from build123d import *

# Parameters (mm, degrees)
SKETCH1_R           = 5
BOSS_EXTRUDE1_DEPTH = 20
SKETCH2_R           = 5
CUT_EXTRUDE1_DEPTH  = 75
SKETCH3_R           = 22.485447426
BOSS_EXTRUDE2_DEPTH = 3.5
SKETCH4_R           = 20.327044556
BOSS_EXTRUDE3_DEPTH = 5.5
SKETCH5_R           = 18.043078954
SKETCH5_R_2         = 5.853514337
CUT_EXTRUDE2_DEPTH  = 2
BOSS_EXTRUDE5_START = 25
SKETCH7_R           = 5.853514337
BOSS_EXTRUDE5_DEPTH = 25


with BuildPart() as part:
    # Sketch1 → Boss-Extrude1 (new body)
    with BuildSketch(Plane(origin=(0, 0, 0), x_dir=(1, 0, 0), z_dir=(0, 1, 0))):
        with BuildLine():
            Line((9.177252883, 11.533668593), (42.143741373, -0.928512909))
            ThreePointArc((42.143741373, -0.928512909), (70.658147952, -5.539619318), (42.614104982, -12.458097383))
            Line((42.614104982, -12.458097383), (7.783972854, -12.458097383))
            ThreePointArc((7.783972854, -12.458097383), (-1.224173666, -20.477404202), (-9.243480486, -11.469257682))
            Line((-9.243480486, -11.469257682), (-23.565055604, -11.469257682))
            ThreePointArc((-23.565055604, -11.469257682), (-58.758292474, 4.433528189), (-20.995467888, 12.522508294))
            Line((-20.995467888, 12.522508294), (-7.850200457, 12.522508294))
            ThreePointArc((-7.850200457, 12.522508294), (1.157946064, 20.541815114), (9.177252883, 11.533668593))
        make_face()
        with Locations(Location((0.663526213, 12.028088444, 0), (0, 0, 270))):
            Circle(SKETCH1_R, mode=Mode.SUBTRACT)
        with Locations(Location((-0.729753816, -11.963677532, 0), (0, 0, 270))):
            Circle(SKETCH1_R, mode=Mode.SUBTRACT)
    extrude(amount=BOSS_EXTRUDE1_DEPTH)

    # Sketch2 → Cut-Extrude1 (cut)
    with BuildSketch(Plane(origin=(0, 20, 0), x_dir=(1, 0, 0), z_dir=(0, 1, 0))):
        with Locations(Location((55.93095175, -6.140433438, 0), (0, 0, 270))):
            Circle(SKETCH2_R)
    extrude(amount=-CUT_EXTRUDE1_DEPTH, mode=Mode.SUBTRACT)

    # Sketch3 → Boss-Extrude2 (add)
    with BuildSketch(Plane.XZ):
        with Locations(Location((-38.546840471, -2.268823063, 0), (0, 0, 37.660146308))):
            Circle(SKETCH3_R)
    extrude(amount=BOSS_EXTRUDE2_DEPTH)

    # Sketch4 → Boss-Extrude3 (add)
    with BuildSketch(Plane(origin=(0, 20, 0), x_dir=(1, 0, 0), z_dir=(0, 1, 0))):
        with Locations(Location((-38.546840471, 2.268823063, 0), (0, 0, 30.293894425))):
            Circle(SKETCH4_R)
    extrude(amount=BOSS_EXTRUDE3_DEPTH)

    # Sketch5 → Cut-Extrude2 (cut)
    with BuildSketch(Plane.XZ.offset(3.5)):
        with Locations(Location((-38.546840471, -2.268823063, 0), (0, 0, 270))):
            Circle(SKETCH5_R)
        with Locations(Location((-38.546840471, -2.268823063, 0), (0, 0, 270))):
            Circle(SKETCH5_R_2, mode=Mode.SUBTRACT)
    extrude(amount=-CUT_EXTRUDE2_DEPTH, mode=Mode.SUBTRACT)

    # Sketch7 → Boss-Extrude5 (add)
    with BuildSketch(Plane.XZ.offset(3.5).offset(BOSS_EXTRUDE5_START)):
        with Locations(Location((-38.546840471, -2.268823063, 0), (0, 0, 270))):
            Circle(SKETCH7_R)
    extrude(amount=-BOSS_EXTRUDE5_DEPTH)


solid = part.part
The model under review builds one solid part; all positions refer to its coordinate system, in mm. A direction names the side the tool comes from. Round coordinates to 2 decimals unless told otherwise and drop trailing zeros. Order: outer loops, then holes, each group sorted by start corner. A loop starts at its lowest first (then second) coordinate and runs counter-clockwise, first axis right, second up. Notation, with made-up numbers: (77, -0.75) -> (109, -0.75) arc R10 cw to (109, 3.25) -> close; hole circle Ø3 at (22.5, 84). An arc over 180 degrees is marked (long way). Use CSV: the item, a comma, the result in double quotes. Start each with the question number.
(1) Tool access review of faces 5 (the face through (-59.003, 0, -3.196)), 6 (the face through (-56.16, -2.51, 1.64)), 7 (the face through (-15, 10, -12.523)): name each direction out of +Z, -Z, +X, -X, +Y, -Y from which nothing blocks a thin tool from reaching the whole face with its end or side.
(2) Consider section B-B on x = -27.5. Write out the cut boundary in (y, z).
(3) Wall thickness on probe 1 along X at (y, z) = (13, 12); probe 2 along Y at (x, z) = (-54, 2); probe 3 along Z at (x, y) = (-11.5, 18): over which ranges is each line inside the solid? List them lowest first. Write a range as from..to.
(4) Mouldability with a two-part tool opening along X and no side actions: class faces 1 (the face through (25.4, 9.9, -5.4)), 2 (the face through (24, 20, 4)), 3 (the face through (0.97, 9.86, -20.55)), 4 (the face through (-16.84, -1.73, 3.6)) as pulls with the +X half, pulls with the -X half, needs draft (parallel to the pull), parting line crosses it, or undercut.
(5) Consider section C-C on y = 2. Write out the cut boundary in (x, z).
(6) Consider section A-A on z = -2. Write out the cut boundary in (x, y), and give its area (3 significant figures).
(7) Consider section D-D on y = 22.5. Write out the cut boundary in (x, z).
(8) Insertion check: pin 1 (3 mm diameter, centred on y = 4, z = 9.5, fed in from +X); pin 2 (12.5 mm diameter, centred on x = 7.5, z = -1.5, fed in from +Y); pin 3 (20.5 mm diameter, centred on x = 37, z = -1.5, fed in from -Y). Each pin has a flat end and moves straight along its axis. Give the tip position at first contact, or say it passes through.
Responses:
1,face 5,"+Y"
1,face 6,"-Y"
1,face 7,"-Z, +Y"
2,outline,"(-3.5, -21.85) -> (0, -21.85) -> (0, -19.33) -> (25.5, -19.33) -> (25.5, 14.79) -> (0, 14.79) -> (0, 17.32) -> (-3.5, 17.32) -> (-3.5, 12) -> (-1.5, 12) -> (-1.5, -16.53) -> (-3.5, -16.53) -> close"
3,probe 1,"-53.02..-24.07, -9.26..-5.73, 4.27..69.46"
3,probe 2,"-1.5..25.5"
3,probe 3,"-12.52..11.47"
4,face 1,"undercut"
4,face 2,"needs draft"
4,face 3,"undercut"
4,face 4,"parting line crosses it"
5,outline,"(-23.57, 11.47) arc R20.33 ccw (long way) to (-21, -12.52) -> (-7.85, -12.52) arc R8.53 ccw to (9.18, -11.53) -> (42.14, 0.93) arc R14.74 ccw (long way) to (42.61, 12.46) -> (7.78, 12.46) arc R8.53 ccw to (-9.24, 11.47) -> close; hole circle Ø10 at (-0.73, 11.96); hole circle Ø10 at (0.66, -12.03); hole circle Ø10 at (55.93, 6.14)"
6,outline,"(-61.03, -3.5) -> (-56.59, -3.5) -> (-56.59, -1.5) -> (-44.39, -1.5) -> (-44.39, -28.5) -> (-32.7, -28.5) -> (-32.7, -1.5) -> (-20.51, -1.5) -> (-20.51, -3.5) -> (-16.06, -3.5) -> (-16.06, 0) -> (34.4, 0) -> (34.4, 20) -> (-18.22, 20) -> (-18.22, 25.5) -> (-58.87, 25.5) -> (-58.87, 0) -> (-61.03, 0) -> close; (43.64, 0) -> (68.22, 0) -> (68.22, 20) -> (43.64, 20) -> close"
6,area,"2,980 mm²"
7,outline,"circle Ø40.65 at (-38.55, -2.27)"
8,pin 1,"x = 70.55"
8,pin 2,"y = 20"
8,pin 3,"y = 0"
